CAD build for the part. Positions are in the model's coordinates, mm. A direction names the side the tool comes from. Round coordinates to 2 decimals unless told otherwise and drop trailing zeros. Write each loop counter-clockwise with the first axis right and the second up, starting at its lowest first coordinate (ties: lowest second). Pieces come first, ordered by that corner, then holes. Notation, with made-up numbers: (-34.75, 0.25) -> (22.25, 0.25) arc R17 cw to (22.25, 26.25) -> close; hole circle Ø9 at (31.25, 70). An arc over 180 degrees is marked (long way). Answer in a Markdown table with one row per item. Add a question column.
Autodesk Fusion 360 part; units mm, degrees
sketch "Facade" plane through (0, 0, 0) normal (0, 0, 1) x (1, 0, 0)
  line L0 (150, -200) -> (-150, -200)
  line L1 (-150, -200) -> (-150, 200)
  line L2 (-150, 200) -> (150, 200)
  line L3 (150, 200) -> (150, -200)
  line L4 (150, -200) -> (-150, 200) construction
  line L5 (-150, -200) -> (150, 200) construction
  dimension "d4" = 400
  dimension "d5" = 300
sketch "Sketch2" plane through (0, 0, 0) normal (1, 0, 0) x (0, 1, 0)
  line L0 (199.9, 0) -> (199.9, -4.5)
  line L1 (199.9, -4.5) -> (184.4, -4.5)
  line L2 (184.4, -4.5) -> (184.4, -19.8)
  line L3 (184.4, -19.8) -> (182.9, -19.8)
  line L4 (182.9, -19.8) -> (182.9, -3)
  line L5 (182.9, -3) -> (196.9, -3)
  line L6 (196.9, -3) -> (196.9, 0)
  line L7 (199.9, 0) -> (196.9, 0)
  point P0 (200, 0)
  dimension "Gap" = 0.1
  dimension "d7" = 3
  dimension "d8" = 1.5
  dimension "d9" = 14
  dimension "d10" = 19.8
  dimension "d11" = 3
  dimension "d13" = 1.5
extrude "Extrude1" add sketch "Sketch2" along normal mid plane 300 makes body 1
sketch "Sketch4" plane through (0, 0, 0) normal (1, 0, 0) x (0, 1, 0)
  line L0 (188.9002, -10.3) -> (164.1797, -10.3)
  line L1 (184.4, -19.8) -> (182.9, -19.8)
  line L2 (182.9, -11.05) -> (180.4, -11.05)
  line L3 (180.4, -11.05) -> (180.4, -11.625)
  line L4 (180.4, -11.625) -> (177.9, -11.05)
  line L5 (177.9, -11.05) -> (177.9, -11.625)
  line L6 (177.9, -11.625) -> (175.4, -11.05)
  line L7 (175.4, -11.05) -> (175.4, -11.625)
  line L8 (175.4, -11.625) -> (172.9, -11.05)
  line L9 (172.9, -11.05) -> (172.9, -10.3)
  line L10 (180.4, -9.55) -> (180.4, -8.975)
  line L11 (175.4, -8.975) -> (172.9, -9.55)
  line L12 (177.9, -9.55) -> (177.9, -8.975)
  line L13 (180.4, -8.975) -> (177.9, -9.55)
  line L14 (175.4, -9.55) -> (175.4, -8.975)
  line L15 (182.9, -9.55) -> (180.4, -9.55)
  line L16 (177.9, -8.975) -> (175.4, -9.55)
  line L17 (172.9, -9.55) -> (172.9, -10.3)
  line L18 (182.9, -19.8) -> (182.9, -3)
  dimension "d26" = 9.5
  dimension "d27" = 1.5
  dimension "d28" = 2.65
  dimension "d29" = 2.5
  dimension "d30" = 2.5
extrude "Extrude2" add sketch "Sketch4" along normal mid plane 228 bodies 1
fillet "Fillet1" radius 2 1 edges at (0, 199.9, -4.5) on bodies 1
sketch "Sketch5" plane through (0, 0, 0) normal (1, 0, 0) x (0, 1, 0)
  line L0 (200, -19) -> (182.9, -19)
  line L1 (182.9, -19) -> (182.9, -3)
  line L2 (182.9, -3) -> (200, -3)
  line L3 (200, -3) -> (200, -19)
  line L4 (182.9, -19.8) -> (182.9, -3)
  line L5 (182.9, -3) -> (196.9, -3)
  line L6 (-200, 0) -> (200, 0)
  line L7 (200, -3) -> (196.9, -3)
  line L8 (196.9, -3) -> (196.9, 0)
  line L9 (196.9, 0) -> (200, 0)
  line L10 (200, 0) -> (200, -3)
  line L11 (196.9, -3) -> (196.9, 0)
  point P0 (200, 0)
  dimension "FacadeThickness" = 19
extrude "Extrude3" add sketch "Sketch5" along normal mid plane 300 separate body makes body 2
sketch "Sketch6" plane through (0, 0, 0) normal (1, 0, 0) x (0, 1, 0)
  line L0 (171.9, -9.3) -> (182.9, -9.3)
  line L1 (182.9, -9.3) -> (182.9, -11.3)
  line L2 (182.9, -11.3) -> (171.9, -11.3)
  line L3 (171.9, -11.3) -> (171.9, -9.3)
  line L4 (171.9, -9.3) -> (182.9, -11.3) construction
  line L5 (182.9, -9.3) -> (171.9, -11.3) construction
  line L6 (172.9, -11.05) -> (172.9, -9.55)
  line L7 (182.9, -19) -> (182.9, -3)
  point P0 (177.4, -10.3)
  point P1 (172.9, -10.3)
  dimension "d39" = 2
  dimension "d40" = 1
extrude "Extrude4" add sketch "Sketch6" along normal mid plane 298 bodies 2
extrude "Extrude5" add 1 faces at (-150, 193.2667, -13.6667) along direction (-1, 0, 0) blind 0.01 on bodies 2 bodies 2
extrude "Extrude6" add 1 faces at (150, 193.2667, -13.6667) along direction (1, 0, 0) blind 0.01 on bodies 2 bodies 2
hidden bodies 2
equation "FacadeWidth = 300 mm"
equation "FacadeHeight = 400 mm"
equation "Shortening = 36 mm"
equation "d4 = FacadeHeight"
equation "d5 = FacadeWidth"
equation "d8 = Thickness"
equation "Thickness = 1.5 mm"
equation "d13 = Thickness"
equation "d24 = FacadeWidth"
equation "d30 = d29"
equation "d31 = FacadeWidth - Shortening * 2"
equation "d37 = FacadeWidth"
equation "d41 = FacadeWidth - 2 mm"
properties part number "Hafele 126.35.945"
Item 1: Saw through at B-B on y = 189.5. Give the cut face in (x, z), then the cut area to 3 significant figures.
Item 2: Saw through at A-A on x = 119. Give the cut face in (y, z).
Item 3: Saw through at C-C on x = -105.5. Give the cut face in (y, z) (3 decimals), then the cut area to 3 significant figures.
Item 4: Pin check, flat tips, straight feed: pin 1 (7 mm diameter, centred on x = -37, y = 190, fed in from -Z); pin 2 (0.6 mm diameter, centred on x = -50.5, z = -9.5, fed in from +Y); pin 3 (2 mm diameter, centred on y = 178.5, z = -10.5, fed in from +X). Stop position of each tip, or through.
Item 5: Tool access for faces 1 (the flat face through (150, 189, -4)), 2 (the flat face through (-2, 191, -4.5)), 3 (the flat face through (-2, 190, -3)): list every direction of +Z, -Z, +X, -X, +Y, -Y with a clear straight run to the whole face (end or side of a thin tool).
Item 6: Drill centre lines: probe 1 along Y at (x, z) = (-6.5, -12); probe 2 along Z at (x, y) = (21.5, 182.75); probe 3 along X at (y, z) = (178.25, -9.75). Where is each one in solid material? Low to high.
Recorded:
| question | item | result |
|---|---|---|
| 1 | outline | (-150, -4.5) -> (150, -4.5) -> (150, -3) -> (-150, -3) -> close |
| 1 | area | 450 mm2 |
| 2 | outline | (182.9, -19.8) -> (184.4, -19.8) -> (184.4, -4.5) -> (197.9, -4.5) arc R2 ccw to (199.9, -2.5) -> (199.9, 0) -> (196.9, 0) -> (196.9, -3) -> (182.9, -3) -> close |
| 3 | outline | (172.9, -11.05) -> (175.4, -11.625) -> (175.4, -11.05) -> (177.9, -11.625) -> (177.9, -11.05) -> (180.4, -11.625) -> (180.4, -11.05) -> (182.9, -11.05) -> (182.9, -19.8) -> (184.4, -19.8) -> (184.4, -4.5) -> (197.9, -4.5) arc R2 ccw to (199.9, -2.5) -> (199.9, 0) -> (196.9, 0) -> (196.9, -3) -> (182.9, -3) -> (182.9, -9.55) -> (180.4, -9.55) -> (180.4, -8.975) -> (177.9, -9.55) -> (177.9, -8.975) -> (175.4, -9.55) -> (175.4, -8.975) -> (172.9, -9.55) -> close |
| 3 | area | 75.9 mm2 |
| 4 | pin 1 | z = -4.5 |
| 4 | pin 2 | y = 184.4 |
| 4 | pin 3 | x = 114 |
| 5 | face 1 | +Z, -Z, +X, +Y, -Y |
| 5 | face 2 | -Z, +X, -X, +Y |
| 5 | face 3 | +Z, +X, -X, -Y |
| 6 | probe 1 | 182.9 to 184.4 |
| 6 | probe 2 | -11.05 to -9.55 |
| 6 | probe 3 | -114 to 114 |
